For this review, take the finished solid that the model builds, in its own axes (mm). A direction names the side the tool comes from. Give positions to 0.01 mm unless a question says otherwise; leave off trailing zeros. Loops run counter-clockwise (first coordinate to the right, second up) from the corner with the lowest first, then second, coordinate; pieces in that order, holes last. Notation, with made-up numbers: M 69,-10 L 96,-10 A17 cw 96,3 Z; hole C 32,6 d5. An arc over 180 degrees is marked long. Use CSV: the item, a comma, the result in double quotes. Start each with the question number.
1. To check wall thickness, follow line 1 (Z direction, x = -408, y = -53.75) (3 decimals); line 2 (X direction, y = -55.75, z = -18.5); line 3 (X direction, y = -54.25, z = -28). State the ranges of each line that lie inside material, in increasing order. Write a range as [from, to].
2. Take a section at A-A, the plane z = -40.5. Write out the cut boundary in (x, y) (1 decimal), and give its area (3 significant figures).
3. Tool access review of faces 1 (the face through (-415, -51, 0)), 2 (the face through (-408.21, -59.77, 1.57)): name each direction out of +Z, -Z, +X, -X, +Y, -Y from which nothing blocks a thin tool from reaching the whole face with its end or side.
4. Insertion check: P1, Ø1.5, axis at y = -52.5, z = -62, coming from the -X side; P2, Ø3, axis at y = -51, z = -51, coming from the +X side; P3, Ø1.5, axis at x = -411, z = -36.5, coming from the -Y side; P4, Ø1, axis at x = -420, z = -61, coming from the +Y side. Each pin has a flat end and moves straight along its axis. Give the tip position at first contact, or say it passes through.
Autodesk Inventor part; units mm, degrees
ref_plane "YZ Plane" through (0, 0, 0) normal (1, 0, 0) x (0, 1, 0)
ref_plane "XZ Plane" through (0, 0, 0) normal (0, 1, 0) x (-1, 0, 0)
ref_plane "XY Plane" through (0, 0, 0) normal (0, 0, 1) x (1, 0, 0)
sketch "Sketch1" plane through (0, 0, 0) normal (0, 0, 1) x (1, 0, 0)
  circle A0 centre (-414.4261, -56.251) radius 4.7625
  point P0 (0, 0)
  dimension "d0" = 9.525
extrude "Extrusion1" add sketch "Sketch1" against normal blind 127
sketch "Sketch2" plane through (-414.4261, -56.251, 0) normal (0, 0, 1) x (1, 0, 0)
  circle A0 centre (0, 0) radius 4.7625
  line L0 (-8.2489, 0) -> (-4.1244, 7.1437)
  line L1 (-4.1244, 7.1437) -> (4.1244, 7.1438)
  line L2 (4.1244, 7.1438) -> (8.2489, 0)
  line L3 (8.2489, 0) -> (4.1244, -7.1437)
  line L4 (4.1244, -7.1437) -> (-4.1244, -7.1438)
  line L5 (-4.1244, -7.1438) -> (-8.2489, 0)
  point P0 (414.4261, 56.251)
  dimension "d3" = 14.2875
extrude "Extrusion2" add sketch "Sketch2" along normal blind 3.175 contours A0 | L0 L1 L2 L3 L4 L5
thread "Thread1"
chamfer "Chamfer1" distance 0.508 angle 45 1 edges at (-419.1886, -56.251, -127)
properties part number "375 bolt x4" material "Steel"
Result set:
1,line 1,"[0, 3.175]"
1,line 2,"[-419.16, -409.69]"
1,line 3,"[-418.75, -410.1]"
2,outline,"C -414.4,-56.3 d9.5"
2,area,"71.3 mm2"
3,face 1,"-Z"
3,face 2,"+Z, -Z, +X, -Y"
4,P1,"x = -418.12"
4,P2,"x = -411.49"
4,P3,"y = -60.19"
4,P4,"through"
